CAD build for the part. Positions are in the model's coordinates, mm. A direction names the side the tool comes from. Round coordinates to 2 decimals unless told otherwise and drop trailing zeros. Order: outer loops, then holes, each group sorted by start corner. A loop starts at its lowest first (then second) coordinate and runs counter-clockwise, first axis right, second up. Notation, with made-up numbers: M 22,-15 L 29,-15 A31 ccw 29,24 Z; hole C 65,31.5 d2. An arc over 180 degrees is marked long. Answer as CSV lines item,"result". Start each with the question number.
```python
from build123d import *

# Parameters (mm, degrees)
SKETCH1_W                 = 4.826
SKETCH1_H                 = 7.9375
BOSS_EXTRUDE1_DEPTH       = 9.525
SKETCH2_W                 = 4.826
SKETCH2_H                 = 4.8895
CUT_EXTRUDE1_DEPTH        = 7.9375
F_6_32_TAPPED_HOLE1_D     = 2.7051
F_6_32_TAPPED_HOLE1_DEPTH = 9.398


with BuildPart() as part:
    # Sketch1 → Boss-Extrude1 (new body)
    with BuildSketch(Plane(origin=(0, 0, 0), x_dir=(1, 0, 0), z_dir=(0, 1, 0))):
        Rectangle(SKETCH1_W, SKETCH1_H)
    extrude(amount=BOSS_EXTRUDE1_DEPTH)

    # Sketch2 → Cut-Extrude1 (cut)
    with BuildSketch(Plane(origin=(0, 9.525, 0), x_dir=(1, 0, 0), z_dir=(0, 1, 0))):
        Rectangle(SKETCH2_W, SKETCH2_H)
    extrude(amount=-CUT_EXTRUDE1_DEPTH, mode=Mode.SUBTRACT)

    # #6-32 Tapped Hole1
    with Locations(Plane.XY.offset(3.96875)):
        with Locations((0, 7.14375)):
            Hole(F_6_32_TAPPED_HOLE1_D / 2, depth=F_6_32_TAPPED_HOLE1_DEPTH)


solid = part.part
```
Q1. Tool access for faces 4 (the cylindrical face through (0.293, 5.823, 3.196)), 5 (the flat face through (0, 1.588, 0)): list every direction of +Z, -Z, +X, -X, +Y, -Y with a clear straight run to the whole face (end or side of a thin tool).
Q2. Band-saw the part on A-A, the plane y = 5.5. Write the cut outline in (x, z), then the cut area to 3 significant figures.
Q3. Band-saw the part on D-D, the plane x = -1.95. Write the cut outline in (y, z) (1 decimal), then the cut area to 3 significant figures.
Q4. Band-saw the part on C-C, the plane y = 7.5. Write the cut outline in (x, z).
Q5. Probe line 1 along Z through (x, y) = (1.6, 9.25); line 2 along Y through (x, z) = (0, -2.95) (3 decimals); line 3 along Y through (x, z) = (-0.3, 0). List the from-to ranges inside material, lowest first. Write a range as from..to.
Q6. Mould opens along Z. For faces 1 (the flat face through (0, 9.525, 3)), 2 (the flat face through (0, 5, -3.969)), 3 (the flat face through (0, 5.6, -2.445)) say: +Z half, -Z half, draft (parallel to the pull), parting line (faces both ways), or undercut.
Q7. Band-saw the part on B-B, the plane x = 0. Write the cut outline in (y, z) (1 decimal), then the cut area to 3 significant figures.
Answer:
1,face 4,"+Z, -Z"
1,face 5,"+X, -X, +Y"
2,outline,"M -2.41,-3.97 L 2.41,-3.97 L 2.41,-2.44 L -2.41,-2.44 Z; M -2.41,2.44 L 2.41,2.44 L 2.41,3.97 L -2.41,3.97 Z"
2,area,"14.7 mm^2"
3,outline,"M 0,-4 L 9.5,-4 L 9.5,-2.4 L 1.6,-2.4 L 1.6,2.4 L 9.5,2.4 L 9.5,4 L 0,4 Z"
3,area,"36.8 mm^2"
4,outline,"M -2.41,-3.97 L -1.3,-3.97 L -1.3,-2.44 L -2.41,-2.44 Z; M -2.41,2.44 L -1.3,2.44 L -1.3,3.97 L -2.41,3.97 Z; M 1.3,-3.97 L 2.41,-3.97 L 2.41,-2.44 L 1.3,-2.44 Z; M 1.3,2.44 L 2.41,2.44 L 2.41,3.97 L 1.3,3.97 Z"
5,line 1,"z = -3.97..-2.44, 2.44..3.97"
5,line 2,"y = 0..5.791, 8.496..9.525"
5,line 3,"y = 0..1.59"
6,face 1,"draft"
6,face 2,"-Z half"
6,face 3,"undercut"
7,outline,"M 0,-4 L 5.8,-4 L 5.8,-2.4 L 1.6,-2.4 L 1.6,2.4 L 5.8,2.4 L 5.8,4 L 0,4 Z; M 8.5,-4 L 9.5,-4 L 9.5,-2.4 L 8.5,-2.4 Z; M 8.5,2.4 L 9.5,2.4 L 9.5,4 L 8.5,4 Z"
7,area,"28.5 mm^2"
